```python
from build123d import *

# Parameters (mm, degrees)
PAD_DEPTH           = 4.064
POCKET_DEPTH        = 4.064
HOLE_D              = 4.572
HOLE_DEPTH          = 635
HOLE_CBORE_D        = 10.414
HOLE_CBORE_DEPTH    = 1.016
POCKET001_DEPTH     = 4.064
HOLE001_D           = 3.499993
HOLE001_DEPTH       = 635
HOLE001_CSINK_D     = 7.000011
HOLE001_CSINK_ANGLE = 120
SKETCH005_R         = 2.286
POCKET002_DEPTH     = 4.064
PAD001_DEPTH        = 2.032
HOLE002_D           = 4.572
HOLE002_DEPTH       = 635
HOLE002_CBORE_D     = 7.50001
HOLE002_CBORE_DEPTH = 2.032


with BuildPart() as part:
    # Sketch → Pad (new body)
    with BuildSketch(Plane.XY):
        with BuildLine():
            Line((-97.79, 80.01), (-97.79, -80.01))
            ThreePointArc((-97.79, -80.01), (-92.582359, -92.582359), (-80.01, -97.79))
            Line((-80.01, -97.79), (80.01, -97.79))
            ThreePointArc((80.01, -97.79), (92.582359, -92.582359), (97.79, -80.01))
            Line((97.79, -80.01), (97.79, 80.01))
            Line((-97.79, 80.01), (97.79, 80.01))
        make_face()
    extrude(amount=PAD_DEPTH)

    # Sketch001 (on Face8 of Pad) → Pocket (cut)
    with BuildSketch(Plane.XY.offset(4.064)):
        with BuildLine():
            ThreePointArc((-29.858031, 5.035139), (-40.005, -21.59), (-29.858031, -48.215139))
            Line((-29.858031, -48.215139), (-3.232892, -21.59))
            Line((-3.232892, -21.59), (-29.858031, 5.035139))
        make_face()
        with BuildLine():
            ThreePointArc((26.625139, 8.268031), (0, 18.415), (-26.625139, 8.268031))
            Line((-26.625139, 8.268031), (0, -18.357108))
            Line((0, -18.357108), (26.625139, 8.268031))
        make_face()
        with BuildLine():
            ThreePointArc((29.858031, -48.215139), (40.005, -21.59), (29.858031, 5.035139))
            Line((3.232892, -21.59), (29.858031, 5.035139))
            Line((3.232892, -21.59), (29.858031, -48.215139))
        make_face()
        with BuildLine():
            ThreePointArc((-26.625139, -51.448031), (0, -61.595), (26.625139, -51.448031))
            Line((0, -24.822892), (26.625139, -51.448031))
            Line((0, -24.822892), (-26.625139, -51.448031))
        make_face()
    extrude(amount=-POCKET_DEPTH, mode=Mode.SUBTRACT)

    # Hole
    with Locations(Plane.XY.offset(4.064)):
        with Locations((-35.7505, 14.1605), (35.7505, 14.1605), (35.7505, -57.3405), (-35.7505, -57.3405)):
            CounterBoreHole(HOLE_D / 2, HOLE_CBORE_D / 2, HOLE_CBORE_DEPTH, depth=HOLE_DEPTH)

    # Sketch003 (on Face5 of Hole) → Pocket001 (cut)
    with BuildSketch(Plane.XY.offset(4.064)):
        Polygon((-50.8, 80.01), (-50.8, 34.29), (-45.72, 34.29), (-45.72, 29.21), (45.72, 29.21), (45.72, 34.29), (50.8, 34.29), (50.8, 80.01), align=None)
    extrude(amount=-POCKET001_DEPTH, mode=Mode.SUBTRACT)

    # Hole001
    with Locations(Plane.XY.offset(4.064)):
        with Locations((-48.26, 31.75), (48.26, 31.75)):
            CounterSinkHole(HOLE001_D / 2, HOLE001_CSINK_D / 2, depth=HOLE001_DEPTH, counter_sink_angle=HOLE001_CSINK_ANGLE)

    # Sketch005 (on Face5 of Hole001) → Pocket002 (cut)
    with BuildSketch(Plane.XY.offset(4.064)):
        with Locations((66.04, 67.31)):
            Circle(SKETCH005_R)
        with Locations((-66.04, 67.31)):
            Circle(SKETCH005_R)
    extrude(amount=-POCKET002_DEPTH, mode=Mode.SUBTRACT)

    # Sketch006 (on Face5 of Pocket002) → Pad001 (join)
    with BuildSketch(Plane.XY.offset(4.064)):
        with BuildLine():
            Line((-97.79, 80.01), (-80.01, 80.01))
            Line((-80.01, 80.01), (-80.01, -62.23))
            ThreePointArc((-62.23, -80.01), (-67.437641, -67.437641), (-80.01, -62.23))
            Line((-62.23, -80.01), (62.23, -80.01))
            ThreePointArc((80.01, -62.23), (67.437641, -67.437641), (62.23, -80.01))
            Line((80.01, -62.23), (80.01, 80.01))
            Line((80.01, 80.01), (97.79, 80.01))
            Line((97.79, 80.01), (97.79, -80.01))
            ThreePointArc((80.01, -97.79), (92.582359, -92.582359), (97.79, -80.01))
            Line((80.01, -97.79), (-80.01, -97.79))
            ThreePointArc((-97.79, -80.01), (-92.582359, -92.582359), (-80.01, -97.79))
            Line((-97.79, -80.01), (-97.79, 80.01))
        make_face()
    extrude(amount=PAD001_DEPTH)

    # Hole002
    with Locations(Plane.XY.offset(6.096)):
        with Locations((-91.44, 54.61), (-91.44, -54.61), (-41.91, -92.71), (41.91, -92.71), (91.44, -54.61), (91.44, 54.61)):
            CounterBoreHole(HOLE002_D / 2, HOLE002_CBORE_D / 2, HOLE002_CBORE_DEPTH, depth=HOLE002_DEPTH)


solid = part.part
```
For this review, take the finished solid that the model builds, in its own axes (mm). A direction names the side the tool comes from. Round coordinates to 2 decimals unless told otherwise and drop trailing zeros. Write each loop counter-clockwise with the first axis right and the second up, starting at its lowest first coordinate (ties: lowest second). Pieces come first, ordered by that corner, then holes. Notation, with made-up numbers: M 87.25,83 L 146.25,83 A20 ccw 146.25,106 Z; hole C -26.75,65.25 d6. An arc over 180 degrees is marked long. One line per item, written item: value. Start each with the question number.
(1) We need section D-D (z = 1.5). Count the separate pieces of the cut face and the enclosed holes in it, and give its area (3 significant figures).
(2) Wall thickness on line 1 (X direction, y = 31.75, z = 2.2); line 2 (Y direction, x = -42.5, z = 5); line 3 (X direction, y = 46.5, z = 1.25): over which ranges is each line inside the solid? List them lowest first.
(3) Insertion check: pin 1 (4 mm diameter, centred on x = -66.04, y = 67.31, fed in from +Z); pin 2 (6 mm diameter, centred on x = 41.91, y = -92.71, fed in from +Z); pin 3 (5 mm diameter, centred on x = -37, y = -55.5, fed in from +Z); pin 4 (1.2 mm diameter, centred on x = -48.5, z = 2, fed in from +Y). Each pin has a flat end and moves straight along its axis. Give the tip position at first contact, or say it passes through.
(4) The part is to be moulded in two halves that separate along Y. For faces 4 (the flat face through (97.79, 1, 3)), 5 (the flat face through (-33.5, 13.1, 3.048)), 6 (the flat face through (-48, 34.29, 2)), say which applies: released by +Y, released by -Y, zero draft, split by the parting line, or undercut.
(5) We need section C-C (x = -21). Give the boundary of the cut face in (y, z), and give its area (3 significant figures).
(6) We need section A-A (x = 24). Give the boundary of the cut face in (y, z), and give its area (3 significant figures).
(7) Machinability: for faces 1 (the flat face through (-16.359, -8.464, 2.06)), 2 (the flat face through (8, -81, 6.096)), 3 (the cylindrical face through (30.55, 14.39, 3.56)), which of the approach directions +Z, -Z, +X, -X, +Y, -Y give a long, thin tool a straight path to every point of the face, cutting with its end or side? Answer none if there is none.
(8) We need section B-B (x = 66.04). Give the boundary of the cut face in (y, z), and give its area (3 significant figures).
Result:
1. separate pieces: 1
1. enclosed holes: 18
1. area: 25,000 mm²
2. line 1: -97.79 to -50.01, -46.51 to -45.72, 45.72 to 46.51, 50.01 to 97.79
2. line 2: -97.79 to -96.41, -89.01 to -80.01
2. line 3: -97.79 to -50.8, 50.8 to 97.79
3. pin 1: through
3. pin 2: z = 4.06
3. pin 3: z = 3.05
3. pin 4: y = 34.29
4. face 4: zero draft
4. face 5: undercut
4. face 6: released by +Y
5. outline: M -97.79,0 L -55.64,0 L -55.64,4.06 L -80.01,4.06 L -80.01,6.1 L -97.79,6.1 Z; M -45.82,0 L -39.36,0 L -39.36,4.06 L -45.82,4.06 Z; M -3.82,0 L 2.64,0 L 2.64,4.06 L -3.82,4.06 Z; M 12.46,0 L 29.21,0 L 29.21,4.06 L 12.46,4.06 Z
5. area: 328 mm²
6. outline: M -97.79,0 L -53.6,0 L -53.6,4.06 L -80.01,4.06 L -80.01,6.1 L -97.79,6.1 Z; M -48.82,0 L -42.36,0 L -42.36,4.06 L -48.82,4.06 Z; M -0.82,0 L 5.64,0 L 5.64,4.06 L -0.82,4.06 Z; M 10.42,0 L 29.21,0 L 29.21,4.06 L 10.42,4.06 Z
6. area: 345 mm²
7. face 1: +Z, -Z
7. face 2: +Z, +X, -X, +Y, -Y
7. face 3: +Z
8. outline: M -97.79,0 L 65.02,0 L 65.02,4.06 L -69.01,4.06 L -69.01,6.1 L -97.79,6.1 Z; M 69.6,0 L 80.01,0 L 80.01,4.06 L 69.6,4.06 Z
8. area: 762 mm²
